Design review of the part shown in the three views and the two pictorial views. Dimensions are in mm from the part's minimum x, y and z. A direction names the side the tool comes from. Give positions to 0.01 mm unless a question says otherwise; leave off trailing zeros. Order: outer loops, then holes, each group sorted by start corner. A loop starts at its lowest first (then second) coordinate and runs counter-clockwise, first axis right, second up. Notation, with made-up numbers: (-18, -21) - (-1, -21) arc R28 cw to (-1, 8) - close; hole circle Ø7 at (14.5, 35). An arc over 180 degrees is marked (long way). Put each result on its own line as item: value.
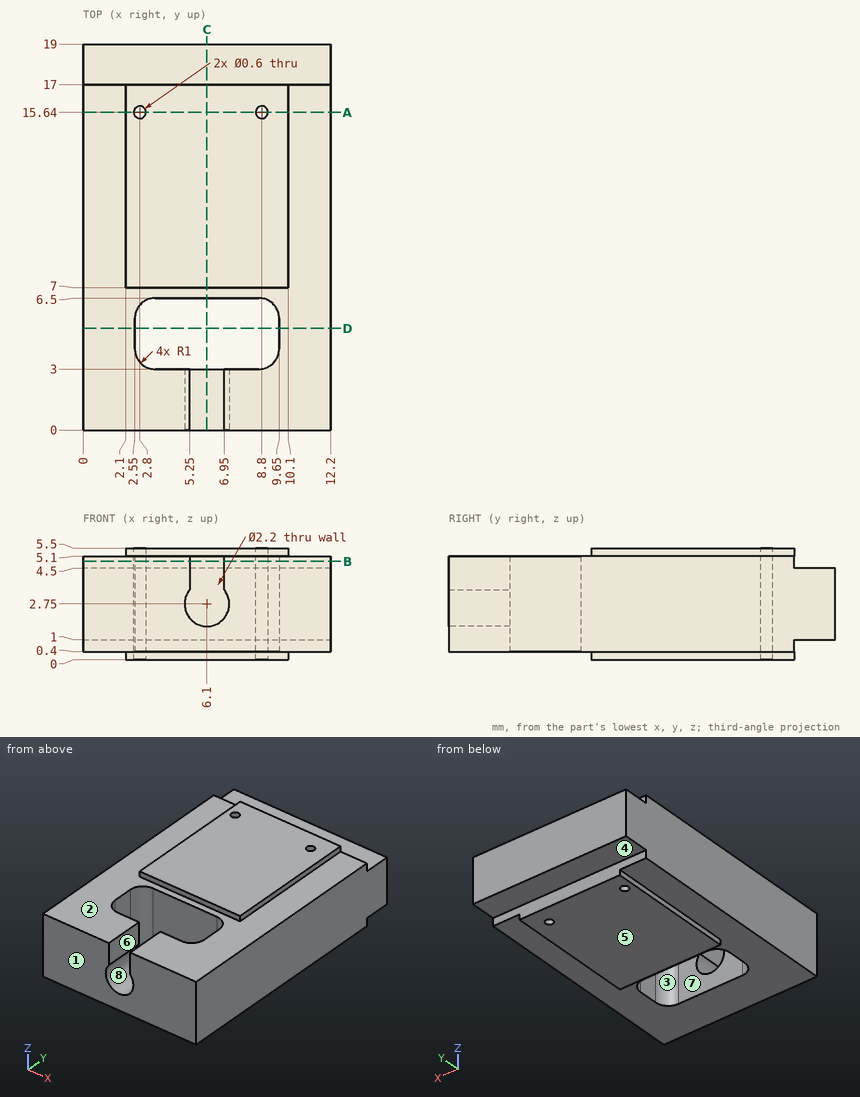
(1) Clearance check with flat-ended pins moving along their axes: pin 1 Ø3 at (x, y) = (1.5, 5.5) entering from +Z; pin 2 Ø1.6 at (x, y) = (5, 17.5) entering from +Z; pin 3 Ø0.8 at (x, z) = (6, 5) entering from +Y. State where each tip first meets the part, or that it passes through.
The answers:
pin 1: z = 5.1
pin 2: z = 5.5
pin 3: y = 17
(2) For the marked faces 4, 5, 6, 7 and 8, list the 3-axis set-ups (+Z, -Z, +X, -X, +Y, -Y) from which the entire face can be reached by the end or side of a thin tool; tool diameter is ignored.
The answers:
face 4: -Z, +X, -X, +Y
face 5: -Z, +X, -X, +Y, -Y
face 6: +Z, -Y
face 7: +Z, -Z
face 8: -Y
(3) Take a section at A-A, the plane y = 15.64. Write out the cut boundary in (x, z), then the cut area to 3 significant figures.
The answers:
outline: (0, 0.4) - (2.1, 0.4) - (2.1, 0) - (2.5, 0) - (2.5, 5.5) - (2.1, 5.5) - (2.1, 5.1) - (0, 5.1) - close; (3.1, 0) - (8.5, 0) - (8.5, 5.5) - (3.1, 5.5) - close; (9.1, 0) - (10.1, 0) - (10.1, 0.4) - (12.2, 0.4) - (12.2, 5.1) - (10.1, 5.1) - (10.1, 5.5) - (9.1, 5.5) - close
area: 57.1 mm^2
(4) Take a section at C-C, the plane x = 6.1. Write out the cut boundary in (y, z), then the cut area to 3 significant figures.
The answers:
outline: (0, 0.4) - (3, 0.4) - (3, 1.65) - (0, 1.65) - close; (6.5, 0.4) - (7, 0.4) - (7, 0) - (17, 0) - (17, 1) - (19, 1) - (19, 4.5) - (17, 4.5) - (17, 5.5) - (7, 5.5) - (7, 5.1) - (6.5, 5.1) - close
area: 68.1 mm^2
(5) The part is to be moulded in two halves that separate along Y. For the marked faces 1, 2 and 3, say which applies: pulls with the +Y half, pulls with the -Y half, needs draft (parallel to the pull), parting line crosses it, or undercut.
The answers:
face 1: pulls with the -Y half
face 2: needs draft
face 3: undercut
(6) Wall thickness on L1, parallel to Y at x = 8.75, z = 5; L2, parallel to X at y = 1.9, z = 2.75; L3, parallel to X at y = 4.5, z = 3.5: over which ranges is each line inside the solid? List them lowest first.
The answers:
L1: 0 to 3.01, 6.49 to 15.34, 15.94 to 17
L2: 0 to 5, 7.2 to 12.2
L3: 0 to 2.55, 9.65 to 12.2
(7) Take a section at D-D, the plane y = 5. Write out the cut boundary in (x, z), then the cut area to 3 significant figures.
The answers:
outline: (0, 0.4) - (2.55, 0.4) - (2.55, 5.1) - (0, 5.1) - close; (9.65, 0.4) - (12.2, 0.4) - (12.2, 5.1) - (9.65, 5.1) - close
area: 24.0 mm^2
(8) Take a section at B-B, the plane z = 4.85. Write out the cut boundary in (x, y), then the cut area to 3 significant figures.
The answers:
outline: (0, 0) - (5.25, 0) - (5.25, 3) - (3.55, 3) arc R1 cw to (2.55, 4) - (2.55, 5.5) arc R1 cw to (3.55, 6.5) - (8.65, 6.5) arc R1 cw to (9.65, 5.5) - (9.65, 4) arc R1 cw to (8.65, 3) - (6.95, 3) - (6.95, 0) - (12.2, 0) - (12.2, 17) - (0, 17) - close; hole circle Ø0.6 at (2.8, 15.64); hole circle Ø0.6 at (8.8, 15.64)
area: 178 mm^2
